from build123d import *

# Parameters (mm, degrees)
SZKIC1_R                    = 15
DODANIE_WYCI_GNI_CIE1_DEPTH = 20


with BuildPart() as part:
    # Szkic1 → Dodanie-wyciągnięcie1 (new body)
    with BuildSketch(Plane.XY):
        with BuildLine():
            Line((-5, 65.017468147), (5, 65.017468147))
            Line((5, 65.017468147), (15, 47.696960071))
            ThreePointArc((15, 47.696960071), (19.134171618, 46.193976626), (23.12024219, 44.333445626))
            Line((23.12024219, 44.333445626), (42.438758716, 49.509826528))
            Line((42.438758716, 49.509826528), (49.509826528, 42.438758716))
            Line((49.509826528, 42.438758716), (44.333445626, 23.12024219))
            ThreePointArc((44.333445626, 23.12024219), (46.193976626, 19.134171618), (47.696960071, 15))
            Line((47.696960071, 15), (65.017468147, 5))
            Line((65.017468147, 5), (65.017468147, -5))
            Line((65.017468147, -5), (47.696960071, -15))
            ThreePointArc((47.696960071, -15), (46.193976626, -19.134171618), (44.333445626, -23.12024219))
            Line((44.333445626, -23.12024219), (49.509826528, -42.438758716))
            Line((49.509826528, -42.438758716), (42.438758716, -49.509826528))
            Line((42.438758716, -49.509826528), (23.12024219, -44.333445626))
            ThreePointArc((23.12024219, -44.333445626), (19.134171618, -46.193976626), (15, -47.696960071))
            Line((15, -47.696960071), (5, -65.017468147))
            Line((5, -65.017468147), (-5, -65.017468147))
            Line((-5, -65.017468147), (-15, -47.696960071))
            ThreePointArc((-15, -47.696960071), (-19.134171618, -46.193976626), (-23.12024219, -44.333445626))
            Line((-23.12024219, -44.333445626), (-42.438758716, -49.509826528))
            Line((-42.438758716, -49.509826528), (-49.509826528, -42.438758716))
            Line((-49.509826528, -42.438758716), (-44.333445626, -23.12024219))
            ThreePointArc((-44.333445626, -23.12024219), (-46.193976626, -19.134171618), (-47.696960071, -15))
            Line((-47.696960071, -15), (-65.017468147, -5))
            Line((-65.017468147, -5), (-65.017468147, 5))
            Line((-65.017468147, 5), (-47.696960071, 15))
            ThreePointArc((-47.696960071, 15), (-46.193976626, 19.134171618), (-44.333445626, 23.12024219))
            Line((-44.333445626, 23.12024219), (-49.509826528, 42.438758716))
            Line((-49.509826528, 42.438758716), (-42.438758716, 49.509826528))
            Line((-42.438758716, 49.509826528), (-23.12024219, 44.333445626))
            ThreePointArc((-23.12024219, 44.333445626), (-19.134171618, 46.193976626), (-15, 47.696960071))
            Line((-15, 47.696960071), (-5, 65.017468147))
        make_face()
        Circle(SZKIC1_R, mode=Mode.SUBTRACT)
    extrude(amount=DODANIE_WYCI_GNI_CIE1_DEPTH)


solid = part.part
Model file for the job. Use its own axes, mm. A direction names the side the tool comes from. Give positions to 0.01 mm unless a question says otherwise; leave off trailing zeros. Loops run counter-clockwise (first coordinate to the right, second up) from the corner with the lowest first, then second, coordinate; pieces in that order, holes last.
1) Flat gauge pins, fed straight in: pin 1 Ø4 at (x, z) = (-23.5, 11.5) entering from +Y; pin 2 Ø5 at (y, z) = (-27.5, 13) entering from +X; pin 3 Ø1 at (x, z) = (-20.5, 17) entering from -Y. Where does each tip first touch, or does it go through?
2) Saw through at C-C (x = 1.5). Write the cut outline in (y, z), plus the area to 3 significant figures.
3) Saw through at A-A (y = 0). Write the cut outline in (x, z), plus the area to 3 significant figures.
4) Saw through at D-D (y = -51.5). Write the cut outline in (x, z), plus the area to 3 significant figures.
5) Tool access for faces 5 (the flat face through (32.915, -46.958, 9.86)), 6 (the flat face through (-32.915, 46.958, 9.86)), 7 (the flat face through (-46.958, -32.915, 9.86)): list every direction of +Z, -Z, +X, -X, +Y, -Y with a clear straight run to the whole face (end or side of a thin tool).
6) Pull direction Y, two halves, no side cores. Call faces 1 (the flat face through (46.958, 32.915, 9.86)), 2 (the flat face through (46.885, -32.644, 9.86)), 3 (the flat face through (65.017, 0, 10)), 4 (the flat face through (0, -65.017, 10)): +Y half, -Y half, draft (parallel to the pull), parting line (faces both ways), or undercut.
7) Wall check: line 1 (Y direction, x = 0, z = 6.75); line 2 (Y direction, x = -13, z = 14.5); line 3 (X direction, y = 42, z = 14.25). Give the ranges that are in metal, low to high.
Answer block:
1. pin 1: stops at y = 45.14
1. pin 2: stops at x = 46.18
1. pin 3: stops at y = -45.83
2. outline: (-65.02, 0) - (-14.92, 0) - (-14.92, 20) - (-65.02, 20) - close; (14.92, 0) - (65.02, 0) - (65.02, 20) - (14.92, 20) - close
2. area: 2,000 mm2
3. outline: (-65.02, 0) - (-15, 0) - (-15, 20) - (-65.02, 20) - close; (15, 0) - (65.02, 0) - (65.02, 20) - (15, 20) - close
3. area: 2,000 mm2
4. outline: (-12.8, 0) - (12.8, 0) - (12.8, 20) - (-12.8, 20) - close
4. area: 512 mm2
5. face 5: +Z, -Z, -Y
5. face 6: +Z, -Z, +Y
5. face 7: +Z, -Z, -X
6. face 1: undercut
6. face 2: undercut
6. face 3: draft
6. face 4: -Y half
7. line 1: y = -65.02 to -15, 15 to 65.02
7. line 2: y = -51.16 to -7.48, 7.48 to 51.16
7. line 3: x = -49.39 to 49.39
